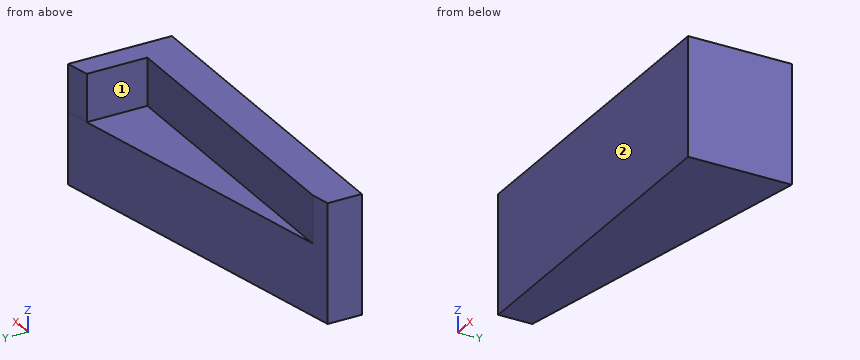
```python
from build123d import *

# Parameters (mm, degrees)
F1_DEPTH  = 15
F3_DEPTH  = 10
F3_FACE_W = 90
F3_FACE_H = 25
F4_DEPTH  = 3
F6_DEPTH  = 25


with BuildPart() as f1:
    # F0 (on Top) → F1 (new body)
    with BuildSketch(Plane.XY):
        Polygon((60, 12.5), (0, 0), (60, 0), align=None)
        Polygon((60, 12.5), (60, 0), (90, 0), (90, 18.75), align=None)
    extrude(amount=F1_DEPTH)

    # F2 (on face) → F3 (join)
    with BuildSketch(Plane.XY.offset(15)):
        Polygon((0, 0), (90, 0), (90, 18.75), (85.000001, 17.708334), (85.000001, 5), (24, 5), align=None)
    extrude(amount=F3_DEPTH)

    # F3_face (on face) → F4 (join)
    with BuildSketch(Plane(origin=(45, 0, 12.5), x_dir=(1, 0, 0), z_dir=(0, -1, 0))):
        Rectangle(F3_FACE_W, F3_FACE_H)
    extrude(amount=F4_DEPTH)

    # F5 (on face) → F6 (cut, through all)
    with BuildSketch(Plane.XY.offset(25)):
        Polygon((0, -3), (20, -3), (20, 4.166667), (0, 0), align=None)
    extrude(amount=-F6_DEPTH, mode=Mode.SUBTRACT)


solid = f1.part
```
The model under review builds one solid part; all positions refer to its coordinate system, in mm. Face numbers are marked on the shaded views. A direction names the side the tool comes from. Give positions to 0.01 mm unless a question says otherwise; leave off trailing zeros. Write each loop counter-clockwise with the first axis right and the second up, starting at its lowest first coordinate (ties: lowest second). Pieces come first, ordered by that corner, then holes.
(1) Consider section C-C, the plane x = 54. Give the boundary of the cut face in (y, z).
(2) Consider section A-A, the plane y = 15.75. Give the boundary of the cut face in (x, z).
(3) To check wall thickness, follow L1, parallel to Y at x = 56, z = 17; L2, parallel to Z at x = 69, y = 13.75; L3, parallel to X at y = 15.5, z = 19.75. State the ranges of each line that lie inside material, in increasing order.
(4) Tool access review of the marked faces 1 and 2: name each direction out of +Z, -Z, +X, -X, +Y, -Y from which nothing blocks a thin tool from reaching the whole face with its end or side.
(5) For P1, Ø3, axis at x = 64.5, y = 16, coming from the +Z side; P2, Ø6, axis at y = 15.5, z = 20.5, coming from the -X side; P3, Ø1.5, axis at x = 71.5, y = 8, coming from the +Z side; P4, Ø1.5, axis at x = 55.5, y = 9.5, coming from the -Z side, all flat-tipped, find the tip position at first contact; note any pin that passes through.
(6) Consider section B-B, the plane z = 18.25. Give the boundary of the cut face in (x, y).
(7) Consider section D-D, the plane z = 8.75. Give the boundary of the cut face in (x, y).
Returned:
1. outline: (-3, 0) - (11.25, 0) - (11.25, 15) - (5, 15) - (5, 25) - (-3, 25) - close
2. outline: (75.6, 0) - (90, 0) - (90, 25) - (85, 25) - (85, 15) - (75.6, 15) - close
3. L1: y = -3 to 5
3. L2: z = 0 to 15
3. L3: x = 85 to 90
4. face 1: +Z, -X, +Y
4. face 2: +Z, -Z, +X, -X, -Y
5. P1: passes through
5. P2: stops at x = 85
5. P3: stops at z = 15
5. P4: stops at z = 0
6. outline: (20, -3) - (90, -3) - (90, 18.75) - (85, 17.71) - (85, 5) - (24, 5) - (20, 4.17) - close
7. outline: (20, -3) - (90, -3) - (90, 18.75) - (20, 4.17) - close
